Study the drawing (mm; zero at the part's minimum x, y, z) and answer. A direction names the side the tool comes from. Round coordinates to 2 decimals unless told otherwise and drop trailing zeros. Write each loop counter-clockwise with the first axis right and the second up, starting at its lowest first coordinate (ties: lowest second). Pieces come first, ordered by that corner, then holes. Notation, with made-up numbers: M 42.5,17.5 L 58.5,17.5 A4 cw 58.5,23.5 Z; hole C 61.25,44.5 d9. An arc over 180 degrees is marked long. Write each question's results on one line, items separated by ' | '.
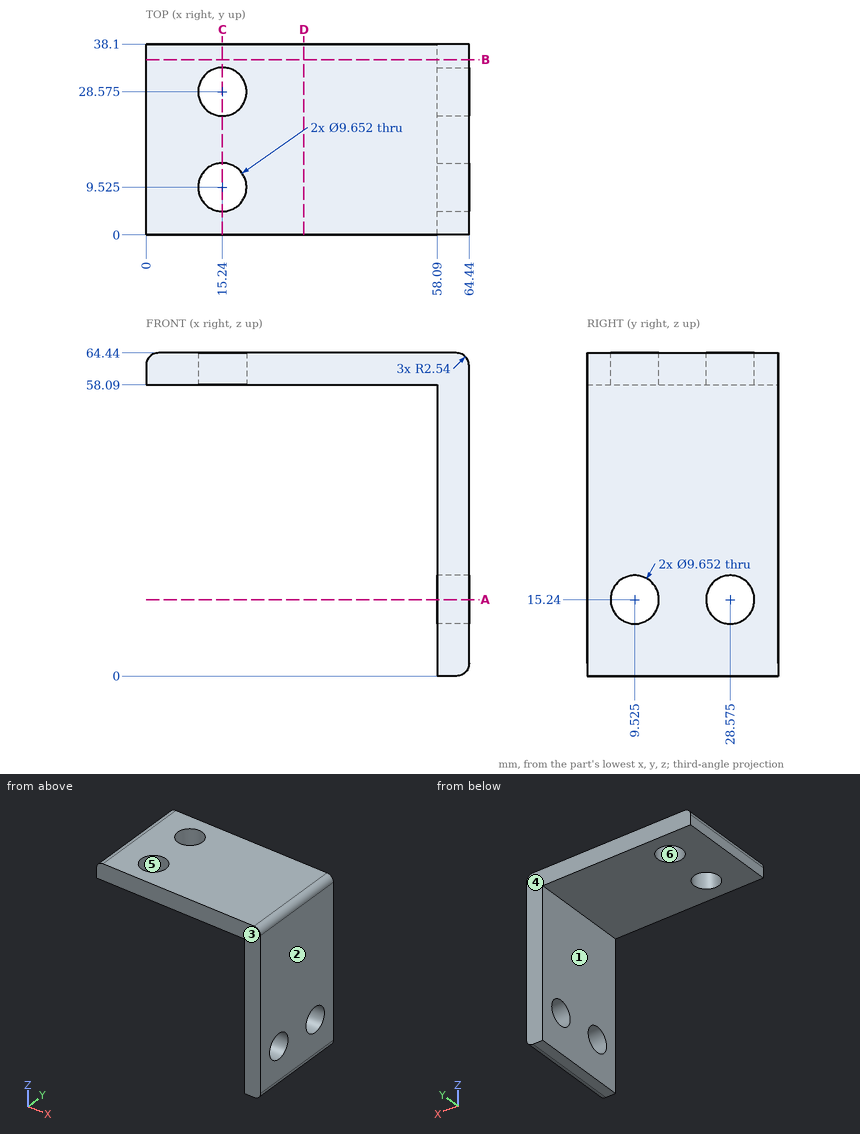
1) Each of these flat-tipped pins is pushed along its axis until it touches: pin 1 (11.5 mm diameter, centred on x = 23.5, y = 24, fed in from -Z); pin 2 (1.5 mm diameter, centred on y = 19, z = 16, fed in from -X). Where does it stop, or does it pass through?
Return value:
pin 1: z = 58.09 | pin 2: x = 58.09
2) The mould has two halves that part along Y. Classify the marked faces 3, 4, 5 and 6: +Y half, -Y half, draft (parallel to the pull), parting line (faces both ways), or undercut.
Return value:
face 3: -Y half | face 4: +Y half | face 5: undercut | face 6: undercut
3) Find the intervals of material crossed by line 1 (Y direction, x = 61.5, z = 15.24); line 2 (Y direction, x = 15, z = 61) (3 decimals); line 3 (X direction, y = 3.5, z = 40.5), in increasing order.
Return value:
line 1: 0 to 4.7, 14.35 to 23.75, 33.4 to 38.1 | line 2: 0 to 4.705, 14.345 to 23.755, 33.395 to 38.1 | line 3: 58.09 to 64.44
4) A tool of negligible diameter and unlimited length cuts with its end or side. For the marked faces 1 and 2, from which of +Z, -Z, +X, -X, +Y, -Y can it reach the whole face along a straight path? Write none if from no direction.
Return value:
face 1: -Z, -X, +Y, -Y | face 2: +Z, -Z, +X, +Y, -Y
5) Section B-B (y = 35) is taken. Determine the outline of the cut face in (x, z), then the cut area to 3 significant figures.
Return value:
outline: M 0,58.09 L 58.09,58.09 L 58.09,0 L 61.9,0 A2.54 ccw 64.44,2.54 L 64.44,61.9 A2.54 ccw 61.9,64.44 L 2.54,64.44 A2.54 ccw 0,61.9 Z | area: 774 mm²
6) Section A-A (z = 15.24) is taken. Determine the outline of the cut face in (x, y), then the cut area to 3 significant figures.
Return value:
outline: M 58.09,0 L 64.44,0 L 64.44,4.7 L 58.09,4.7 Z; M 58.09,14.35 L 64.44,14.35 L 64.44,23.75 L 58.09,23.75 Z; M 58.09,33.4 L 64.44,33.4 L 64.44,38.1 L 58.09,38.1 Z | area: 119 mm²
7) Section D-D (x = 31.5) is taken. Determine the outline of the cut face in (y, z).
Return value:
outline: M 0,58.09 L 38.1,58.09 L 38.1,64.44 L 0,64.44 Z
8) Section C-C (x = 15.24) is taken. Determine the outline of the cut face in (y, z), then the cut area to 3 significant figures.
Return value:
outline: M 0,58.09 L 4.7,58.09 L 4.7,64.44 L 0,64.44 Z; M 14.35,58.09 L 23.75,58.09 L 23.75,64.44 L 14.35,64.44 Z; M 33.4,58.09 L 38.1,58.09 L 38.1,64.44 L 33.4,64.44 Z | area: 119 mm²
